```python
from build123d import *

# Parameters (mm, degrees)
SKETCH_1_W                     = 143
SKETCH_1_H                     = 68
EXTRUDE_1_DEPTH                = 5
HOLE_WIZARD_M2_5_1_D           = 2.9
HOLE_WIZARD_M2_5_1_CSINK_D     = 5.5
HOLE_WIZARD_M2_5_1_CSINK_ANGLE = 90
HOLE_WIZARD_M3_1_D             = 3.4
HOLE_WIZARD_M3_1_CSINK_D       = 6.3
HOLE_WIZARD_M3_1_CSINK_ANGLE   = 90


with BuildPart() as part:
    # 草圖1 → 填料-伸長1 (new body)
    with BuildSketch(Plane(origin=(0, 0, 0), x_dir=(1, 0, 0), z_dir=(0, 1, 0))):
        Rectangle(SKETCH_1_W, SKETCH_1_H)
    extrude(amount=EXTRUDE_1_DEPTH)

    # M2.5 錐坑平頭螺釘的錐孔1 (through all)
    with Locations(Plane(origin=(0, 0, 0), x_dir=(-1, 0, 0), z_dir=(0, -1, 0))):
        with Locations((68, 25), (68, 0), (68, -25)):
            CounterSinkHole(HOLE_WIZARD_M2_5_1_D / 2, HOLE_WIZARD_M2_5_1_CSINK_D / 2, counter_sink_angle=HOLE_WIZARD_M2_5_1_CSINK_ANGLE)

    # M3 錐坑平頭螺釘的錐孔1 (through all)
    with Locations(Plane(origin=(0, 0, 0), x_dir=(-1, 0, 0), z_dir=(0, -1, 0))):
        with Locations((-67.5, 25), (-67.5, 0), (-67.5, -25)):
            CounterSinkHole(HOLE_WIZARD_M3_1_D / 2, HOLE_WIZARD_M3_1_CSINK_D / 2, counter_sink_angle=HOLE_WIZARD_M3_1_CSINK_ANGLE)


solid = part.part
```
Can you work these out from the model? Positions are in its coordinate system, mm. Give positions to 0.01 mm unless a question says otherwise; leave off trailing zeros. Write each loop counter-clockwise with the first axis right and the second up, starting at its lowest first coordinate (ties: lowest second). Pieces come first, ordered by that corner, then holes. Notation, with made-up numbers: (-2.75, 7.5) -> (22.25, 7.5) arc R30 ccw to (22.25, 36.5) -> close; hole circle Ø11 at (-27.5, -3). An arc over 180 degrees is marked (long way). One line per item, written item: value.
Q1. Imagine slicing it at B-B on z = 25. Please give me the cut outline in (x, y), and give its area (3 significant figures).
Results found:
outline: (-71.5, 0) -> (-70.75, 0) -> (-69.45, 1.3) -> (-69.45, 5) -> (-71.5, 5) -> close; (-66.55, 1.3) -> (-65.25, 0) -> (64.35, 0) -> (65.8, 1.45) -> (65.8, 5) -> (-66.55, 5) -> close; (69.2, 1.45) -> (70.65, 0) -> (71.5, 0) -> (71.5, 5) -> (69.2, 5) -> close
area: 680 mm^2
Q2. For P1, Ø3.5, axis at x = -68, z = -25, coming from the -Y side; P2, Ø4.5, axis at x = 67.5, z = 0, coming from the -Y side, each with a flat end and sliding along its axis, tell me the tip position at first contact or that it passes through.
Results found:
P1: stops at y = 1
P2: stops at y = 0.9
Q3. Imagine slicing it at C-C on x = 67.5. Please give me the cut outline in (y, z).
Results found:
outline: (0, -34) -> (5, -34) -> (5, -26.7) -> (1.45, -26.7) -> (0, -28.15) -> close; (0, -21.85) -> (1.45, -23.3) -> (5, -23.3) -> (5, -1.7) -> (1.45, -1.7) -> (0, -3.15) -> close; (0, 3.15) -> (1.45, 1.7) -> (5, 1.7) -> (5, 23.3) -> (1.45, 23.3) -> (0, 21.85) -> close; (0, 28.15) -> (1.45, 26.7) -> (5, 26.7) -> (5, 34) -> (0, 34) -> close
Q4. Please list where these lines run through material, in increasing order: line 1 (Z direction, x = -68, y = 2.75); line 2 (X direction, y = 2.55, z = -25); line 3 (Z direction, x = 67.5, y = 3.15). Write a range as [from, to].
Results found:
line 1: z = [-34, -26.45], [-23.55, -1.45], [1.45, 23.55], [26.45, 34]
line 2: x = [-71.5, -69.45], [-66.55, 65.8], [69.2, 71.5]
line 3: z = [-34, -26.7], [-23.3, -1.7], [1.7, 23.3], [26.7, 34]
Q5. Imagine slicing it at A-A on x = -68. Please give me the cut outline in (y, z).
Results found:
outline: (0, -34) -> (5, -34) -> (5, -26.45) -> (1.3, -26.45) -> (0, -27.75) -> close; (0, -22.25) -> (1.3, -23.55) -> (5, -23.55) -> (5, -1.45) -> (1.3, -1.45) -> (0, -2.75) -> close; (0, 2.75) -> (1.3, 1.45) -> (5, 1.45) -> (5, 23.55) -> (1.3, 23.55) -> (0, 22.25) -> close; (0, 27.75) -> (1.3, 26.45) -> (5, 26.45) -> (5, 34) -> (0, 34) -> close
Q6. We'd pull the mould along X, two halves only. Please class faces 1 (the face through (-69.15, 3.18, 0.88)), 2 (the face through (71.5, 2, 0)), 3 (the face through (-1, 5, 0)): +X half, -X half, draft (parallel to the pull), parting line (faces both ways), or undercut.
Results found:
face 1: undercut
face 2: +X half
face 3: draft
